Autodesk Inventor part; units mm, degrees
ref_plane "YZ Plane" through (0, 0, 0) normal (1, 0, 0) x (0, 1, 0)
ref_plane "XZ Plane" through (0, 0, 0) normal (0, 1, 0) x (-1, 0, 0)
ref_plane "XY Plane" through (0, 0, 0) normal (0, 0, 1) x (1, 0, 0)
sketch "Sketch1" plane through (0, 0, 0) normal (0, 0, 1) x (1, 0, 0)
  line L0 (-9.525, 0) -> (9.525, 0)
  line L1 (9.525, 0) -> (9.525, 44.45)
  line L2 (9.525, 44.45) -> (5.715, 44.45)
  line L3 (5.715, 44.45) -> (4.891, 28.7274)
  line L4 (4.891, 28.7274) -> (-9.525, 28.7274)
  line L5 (-9.525, 28.7274) -> (-9.525, 0)
  point P0 (0, 0)
  point P1 (0, 0)
  dimension "d0" = 44.45
  dimension "d1" = 15.24
  dimension "d2" = 15.7226
  dimension "d3" = 19.05
  dimension "d14" = 93
extrude "Extrusion1" add sketch "Sketch1" along normal mid plane 15.7226
sketch "Sketch2" plane through (0, 0, 0) normal (1, 0, 0) x (0, 1, 0)
  line L0 (-19.05, 9.525) -> (-19.05, -9.525)
  line L1 (-19.05, -9.525) -> (-15.875, -9.525)
  line L2 (-15.875, -9.525) -> (-15.875, -1.5875)
  line L3 (-15.875, -1.5875) -> (-3.175, -1.5875)
  line L4 (-3.175, -1.5875) -> (-3.175, -9.525)
  line L5 (-3.175, -9.525) -> (0, -9.525)
  line L6 (0, -9.525) -> (0, 9.525)
  line L7 (0, 9.525) -> (-3.175, 9.525)
  line L8 (-3.175, 9.525) -> (-3.175, 1.5875)
  line L9 (-3.175, 1.5875) -> (-15.875, 1.5875)
  line L10 (-15.875, 1.5875) -> (-15.875, 9.525)
  line L11 (-15.875, 9.525) -> (-19.05, 9.525)
  line L12 (0, -7.8613) -> (0, 7.8613)
  point P0 (0, 0)
  point P1 (0, 0)
  dimension "d6" = 19.05
  dimension "d7" = 19.05
  dimension "d8" = 3.175
  dimension "d9" = 3.175
extrude "Extrusion2" add sketch "Sketch2" along normal mid plane 19.05
sketch "Sketch6" plane through (0, 0, 7.8613) normal (0, 0, 1) x (1, 0, 0)
  line L0 (4.891, 28.7274) -> (9.525, 28.7274)
  line L1 (9.525, 28.7274) -> (9.525, 44.45)
  line L2 (9.525, 44.45) -> (4.891, 44.45)
  line L3 (4.891, 44.45) -> (4.891, 28.7274)
  point P0 (0, 0)
extrude "Extrusion3" add sketch "Sketch6" against normal blind 15.7226
sketch "Sketch9" plane through (0, 0, 7.8613) normal (0, 0, 1) x (1, 0, 0)
  line L0 (4.891, 44.45) -> (4.891, 28.7274)
  line L1 (-9.525, 28.7274) -> (-9.525, 0)
  line L2 (4.891, 28.7274) -> (-2.729, 28.7274)
  line L3 (4.891, 28.7274) -> (-9.525, 28.7274)
  line L4 (-9.525, 28.7274) -> (-9.525, 26.7462)
  line L5 (-9.525, 26.7462) -> (-2.729, 28.7274)
  point P0 (0, 0)
  dimension "d22" = 14.416
  dimension "d23" = 7.62
  dimension "d24" = 1.9812
extrude "Extrusion5" cut sketch "Sketch9" against normal blind 25.4
fillet "Fillet2" radius 5.08 1 edges at (-2.729, 28.7274, 0)
sketch "Sketch10" plane through (-9.525, -15.875, 1.5875) normal (0, 0, 1) x (1, 0, 0)
  circle A0 centre (9.525, 6.35) radius 0.635
  line L0 (0, 0) -> (0, 12.7)
  line L1 (19.05, -3.175) -> (0, -3.175)
  point P0 (9.525, 15.875)
  dimension "d28" = 9.525
  dimension "d29" = 9.525
  dimension "d30" = 1.27
extrude "Extrusion6" cut sketch "Sketch10" against normal blind 25.4
sketch "Sketch12" plane through (-9.525, -15.875, -1.5875) normal (-1, 0, 0) x (0, 0, 1)
  line L0 (-6.2738, 60.325) -> (-6.2738, 15.875)
  line L1 (9.4488, 42.6212) -> (9.4488, 15.875)
  line L2 (-6.2738, 36.7601) -> (9.4488, 36.7601)
  line L3 (9.4488, 36.7601) -> (9.4488, 19.5053)
  line L4 (9.4488, 19.5053) -> (-6.2738, 19.5053)
  line L5 (-6.2738, 19.5053) -> (-6.2738, 36.7601)
  point P0 (1.5875, 15.875)
extrude "Extrusion7" cut sketch "Sketch12" against normal blind 12.7
sketch "Sketch13" plane through (3.175, -15.875, -1.5875) normal (-1, 0, 0) x (0, 0, 1)
  line L0 (0, 12.7) -> (0, 36.7601)
  line L1 (-6.2738, 36.7601) -> (9.4488, 36.7601)
  line L2 (0, 12.7) -> (0, 0)
  line L3 (3.175, 12.7) -> (3.175, 36.7601)
  line L4 (3.175, 0) -> (3.175, 12.7)
  line L5 (9.4488, 19.5053) -> (-6.2738, 19.5053)
  line L6 (0, 36.7601) -> (3.175, 36.7601)
  line L7 (3.175, 36.7601) -> (3.175, 19.5053)
  line L8 (3.175, 19.5053) -> (0, 19.5053)
  line L9 (0, 19.5053) -> (0, 36.7601)
  point P0 (1.5875, 15.875)
extrude "Extrusion8" add sketch "Sketch13" along normal blind 12.7
sketch "Sketch15" plane through (3.175, 3.6303, 1.5875) normal (0, 0, 1) x (1, 0, 0)
  circle A0 centre (-7.62, 5.0254) radius 0.635
  line L0 (-12.7, 0) -> (-12.7, 17.2548)
  circle A1 centre (-5.715, 9.4248) radius 0.635
  circle A2 centre (-5.08, 14.5048) radius 0.635
  point P0 (-3.175, -3.6303)
  dimension "d40" = 5.08
  dimension "d41" = 1.27
  dimension "d42" = 1.27
  dimension "d45" = 1.27
  dimension "d46" = 6.985
  dimension "d47" = 7.62
extrude "Extrusion9" cut sketch "Sketch15" against normal blind 12.7
sketch "Sketch17" plane through (-9.525, -15.875, -1.5875) normal (-1, 0, 0) x (0, 0, 1)
  line L0 (-7.9375, 15.875) -> (11.1125, 15.875)
  line L1 (0, 19.5053) -> (-3.81, 19.5053)
  line L2 (-3.81, 19.5053) -> (-3.81, 15.875)
  line L3 (-3.81, 15.875) -> (0, 15.875)
  line L4 (0, 15.875) -> (0, 19.5053)
  line L5 (3.175, 19.5053) -> (6.985, 19.5053)
  line L6 (6.985, 19.5053) -> (6.985, 15.875)
  line L7 (6.985, 15.875) -> (3.175, 15.875)
  line L8 (3.175, 15.875) -> (3.175, 19.5053)
  point P0 (1.5875, 15.875)
  dimension "d51" = 3.81
  dimension "d52" = 3.81
extrude "Extrusion10" cut sketch "Sketch17" against normal blind 5.08
sketch "Sketch18" plane through (9.525, 44.45, 7.8613) normal (1, 0, 0) x (0, 0, -1)
  line L0 (-1.6637, -63.5) -> (-1.6637, -60.325)
  line L1 (-1.6637, -60.325) -> (6.2738, -60.325)
  line L2 (6.2738, -60.325) -> (-1.6637, -60.325)
  line L3 (6.2738, -60.325) -> (6.2738, -47.625)
  line L4 (6.2738, -47.625) -> (-1.6637, -47.625)
  line L5 (-1.6637, -47.625) -> (-1.6637, -44.45)
  line L6 (-1.6637, -44.45) -> (-1.6637, -47.625)
  line L7 (-1.6637, -44.45) -> (0, -44.45)
  line L8 (0, -44.45) -> (0, -40.8197)
  line L9 (0, -44.45) -> (0, 0)
  line L10 (15.7226, 0) -> (15.7226, -44.45)
  line L11 (15.7226, -41.3057) -> (15.7226, -44.45)
  line L12 (17.3863, -44.45) -> (15.7226, -44.45)
  line L13 (15.7226, -44.45) -> (17.3863, -44.45)
  line L14 (17.3863, -44.45) -> (17.3863, -47.625)
  line L15 (17.3863, -47.625) -> (17.3863, -44.45)
  line L16 (17.3863, -47.625) -> (9.4488, -47.625)
  line L17 (9.4488, -47.625) -> (9.4488, -60.325)
  line L18 (17.3863, -60.325) -> (9.4488, -60.325)
  line L19 (9.4488, -60.325) -> (17.3863, -60.325)
  line L20 (17.3863, -63.5) -> (17.3863, -60.325)
  line L21 (17.3863, -60.325) -> (17.3863, -63.5)
  line L22 (17.3863, -63.5) -> (-1.6637, -63.5)
  line L23 (-1.6637, -63.5) -> (17.3863, -63.5)
  line L24 (0, -40.8197) -> (15.7226, -40.8197)
  line L25 (9.4488, -40.8197) -> (15.7226, -40.8197)
  line L26 (15.7226, -40.8197) -> (15.7226, -44.45)
  point P0 (7.8613, -44.45)
extrude "Extrusion11" add sketch "Sketch18" along normal blind 6.35
chamfer "Chamfer1" distance 6.35 angle 45 1 edges at (9.525, 3.6303, 0)
sketch "Sketch19" plane through (-9.525, -15.875, -1.5875) normal (0, 0, -1) x (-1, 0, 0)
  circle A0 centre (-9.525, 6.35) radius 0.762
  circle A1 centre (-9.525, 6.35) radius 0.635
  point P0 (-9.525, 15.875)
  dimension "d60" = 0
  dimension "d61" = 0
  dimension "d62" = 1.524
extrude "Extrusion12" cut sketch "Sketch19" against normal blind 6.35
sketch "Sketch20" plane through (3.175, 3.6303, -1.5875) normal (0, 0, -1) x (-1, 0, 0)
  circle A0 centre (5.08, 14.5048) radius 0.762
  circle A1 centre (5.08, 14.5048) radius 0.635
  circle A2 centre (5.715, 9.4248) radius 0.762
  circle A3 centre (5.715, 9.4248) radius 0.635
  circle A4 centre (7.62, 5.0254) radius 0.762
  circle A5 centre (7.62, 5.0254) radius 0.635
  point P0 (3.175, -3.6303)
  dimension "d65" = 0
  dimension "d66" = 0
  dimension "d67" = 1.524
  dimension "d68" = 0
  dimension "d69" = 0
  dimension "d70" = 1.524
  dimension "d71" = 0
  dimension "d72" = 0
  dimension "d73" = 1.524
extrude "Extrusion13" cut sketch "Sketch20" against normal blind 6.35
sketch "Sketch25" plane through (-9.525, -15.875, -1.5875) normal (-1, 0, 0) x (0, 0, 1)
  line L0 (9.4488, 19.5053) -> (9.4488, 15.875)
  line L1 (-6.2738, 15.875) -> (-6.2738, 19.5053)
  line L2 (-6.2738, 15.875) -> (-5.3086, 15.875)
  line L3 (-5.3086, 15.875) -> (-5.3086, 64.7795)
  line L4 (-5.3086, 64.7795) -> (-6.2738, 64.7795)
  line L5 (-6.2738, 64.7795) -> (-6.2738, 15.875)
  line L6 (9.4488, 15.875) -> (8.4836, 15.875)
  line L7 (8.4836, 15.875) -> (8.4836, 64.7795)
  line L8 (8.4836, 64.7795) -> (9.4488, 64.7795)
  line L9 (9.4488, 64.7795) -> (9.4488, 15.875)
  point P0 (1.5875, 15.875)
  dimension "d87" = 15.7226
  dimension "d88" = 0.9652
  dimension "d89" = 0.9652
extrude "Extrusion16" cut sketch "Sketch25" against normal blind 38.1
sketch "Sketch30" plane through (-9.525, 20.8851, 6.8961) normal (0, 0, 1) x (1, 0, 0)
  line L0 (0, 5.8611) -> (0, 0)
  line L1 (14.416, 7.8423) -> (7.5214, 7.8423)
  line L2 (0, 2.9305) -> (8.832, 2.9305)
  line L3 (8.832, 2.9305) -> (8.832, 7.8423)
  line L4 (8.832, 7.8423) -> (0, 7.8423)
  line L5 (0, 7.8423) -> (0, 2.9305)
  point P0 (9.525, -20.8851)
extrude "Extrusion17" add sketch "Sketch30" against normal blind 13.7922
properties part number "mod_gripper_flat" material "Steel, High Strength Low Alloy"
Input: part model. Units: mm. Frame: model coordinates. A direction names the side the tool comes from. Give positions to 0.01 mm unless a question says otherwise; leave off trailing zeros. Loops run counter-clockwise (first coordinate to the right, second up) from the corner with the lowest first, then second, coordinate; pieces in that order, holes last.
1) Line query: L1, parallel to Y at x = 2.75, z = 3 (3 decimals); L2, parallel to Y at x = -7.75, z = -3.5 (3 decimals); L3, parallel to Y at x = -3.75, z = 7 (3 decimals). Output: solid intervals per line, ascending.
A:
L1: y = -19.05 to -15.875, -3.175 to 3.63, 20.885 to 28.727
L2: y = -19.05 to -15.875, -3.175 to 0, 20.885 to 28.727
L3: y = -19.05 to -15.875, -3.175 to 0
2) Mould query, pull axis X, two halves, no side actions, for faces 4 (the flat face through (4.891, 37, 0)), 5 (the flat face through (3, -9, -1.588)), 6 (the cylindrical face through (-3.27, 13.28, -0.02)). Classes: released by +X, released by -X, zero draft, split by the parting line, or undercut.
A:
face 4: released by -X
face 5: zero draft
face 6: undercut
3) Reachability of faces 1 (the flat face through (-7, 0, -4)), 2 (the flat face through (9.525, 27, 0)), 3 (the flat face through (3, -15.875, 6)) from +Z, -Z, +X, -X, +Y, -Y: full face, straight path, thin tool, end or side. Return the list, or none.
A:
face 1: -X
face 2: +Z, -Z, +X, +Y
face 3: +Z, +X, -X
4) Contact query for flat-ended pins moving along their axis: pin 1 (10 mm diameter, centred on y = 10.5, z = -4.5, fed in from +X); pin 2 (2 mm diameter, centred on x = -2, z = -8, fed in from +Y); pin 3 (8 mm diameter, centred on y = 12.5, z = 7, fed in from +X); pin 4 (1.4 mm diameter, centred on x = -2.54, y = 13.06, fed in from -Z). Output: stop coordinate, or through.
A:
pin 1: stops at x = 14
pin 2: stops at y = 0
pin 3: stops at x = 11
pin 4: passes through
5) Section query B-B on z = -8. Return the cut outline in (x, y) (3 decimals).
A:
outline: (-9.525, -19.05) - (15.875, -19.05) - (15.875, -15.875) - (-9.525, -15.875) - close; (-9.525, -3.175) - (15.875, -3.175) - (15.875, 0) - (-9.525, 0) - close
